```python
from build123d import *

# Parameters (mm, degrees)
F0_W     = 558.8
F0_H     = 25.4
F1_DEPTH = 25.4
F2_W     = 558.8
F2_H     = 3.175
F3_DEPTH = 3.175
F5_DEPTH = 25.4
F7_DEPTH = 25.4


with BuildPart() as f1:
    # F0 (on Front) → F1 (new body)
    with BuildSketch(Plane.XZ):
        Rectangle(F0_W, F0_H)
    extrude(amount=F1_DEPTH)

    # F2 (on face) → F3 (cut)
    with BuildSketch(Plane.XY.offset(12.7)):
        with Locations((0, -12.7)):
            Rectangle(F2_W, F2_H)
    extrude(amount=-F3_DEPTH, mode=Mode.SUBTRACT)

    # F4 (on face) → F5 (join)
    with BuildSketch(Plane(origin=(-279.4, 0, 0), x_dir=(0, -1, 0), z_dir=(-1, 0, 0))):
        Polygon((7.9375, -12.7), (17.4625, -12.7), (17.4625, 12.7), (14.2875, 12.7), (14.2875, 9.525), (11.1125, 9.525), (11.1125, 12.7), (7.9375, 12.7), align=None)
    extrude(amount=F5_DEPTH)

    # F6 (on face) → F7 (join)
    with BuildSketch(Plane.YZ.offset(279.4)):
        Polygon((-17.4625, -12.7), (-7.9375, -12.7), (-7.9375, 12.7), (-11.1125, 12.7), (-11.1125, 9.525), (-14.2875, 9.525), (-14.2875, 12.7), (-17.4625, 12.7), align=None)
    extrude(amount=F7_DEPTH)


solid = f1.part
```
Build history of the part. All positions in model axes, mm. A direction names the side the tool comes from. Coordinates: 2 decimals unless noted, no trailing zeros. Order: outer loops, then holes, each group sorted by start corner. A loop starts at its lowest first (then second) coordinate and runs counter-clockwise, first axis right, second up. Notation, with made-up numbers: (73, 72) -> (108, 72) arc R11 ccw to (108, 90) -> close; hole circle Ø7 at (59.25, -38.75). An arc over 180 degrees is marked (long way). Answer in a Markdown table with one row per item. Add a question column.
Q1. Which spindle directions (+Z, -Z, +X, -X, +Y, -Y) get a long thin tool onto all of the face, cutting with end or side? Do faces 1 (the face through (292, -7.938, 0)), 2 (the face through (-292, -7.938, 0)), 3 (the face through (-4, 0, 0)), 4 (the face through (-292, -17.462, 0)), 5 (the face through (292, -17.462, 0)). Say none if no direction does.
Q2. Wall check: line 1 along Y through (x, z) = (262, 10); line 2 along X through (y, z) = (-22.5, -11.25); line 3 along Z through (x, y) = (-6, -13.25) (3 decimals). Give the ranges that are in metal, low to high. Write a range as [from, to].
Q3. Band-saw the part on B-B, the plane z = -2.5. List the corners of the cut face in (x, y), then the cut area to 3 significant figures.
Q4. Band-saw the part on A-A, the plane x = 73.5. List the corners of the cut face in (y, z) (1 decimal).
Q5. Drop flat-ended pins along their axis: pin 1 (4 mm diameter, centred on y = -22, z = -3, fed in from +X); pin 2 (1 mm diameter, centred on x = 87.5, y = -12, fed in from +Z) (3 decimals); pin 3 (4 mm diameter, centred on y = -3, z = -4.5, fed in from -X). Give the stop position or say it passes through.
Answers follow:
| question | item | result |
|---|---|---|
| 1 | face 1 | +Z, -Z, +X, +Y |
| 1 | face 2 | +Z, -Z, -X, +Y |
| 1 | face 3 | +Z, -Z, +X, -X, +Y |
| 1 | face 4 | +Z, -Z, -X, -Y |
| 1 | face 5 | +Z, -Z, +X, -Y |
| 2 | line 1 | [-25.4, -14.29], [-11.11, 0] |
| 2 | line 2 | [-279.4, 279.4] |
| 2 | line 3 | [-12.7, 9.525] |
| 3 | outline | (-304.8, -17.46) -> (-279.4, -17.46) -> (-279.4, -25.4) -> (279.4, -25.4) -> (279.4, -17.46) -> (304.8, -17.46) -> (304.8, -7.94) -> (279.4, -7.94) -> (279.4, 0) -> (-279.4, 0) -> (-279.4, -7.94) -> (-304.8, -7.94) -> close |
| 3 | area | 14,700 mm^2 |
| 4 | outline | (-25.4, -12.7) -> (0, -12.7) -> (0, 12.7) -> (-11.1, 12.7) -> (-11.1, 9.5) -> (-14.3, 9.5) -> (-14.3, 12.7) -> (-25.4, 12.7) -> close |
| 5 | pin 1 | x = 279.4 |
| 5 | pin 2 | z = 9.525 |
| 5 | pin 3 | x = -279.4 |
